The model under review builds one solid part; all positions refer to its coordinate system, in mm. Face numbers are marked on the shaded views. A direction names the side the tool comes from. Coordinates: 2 decimals unless noted, no trailing zeros. Write each loop counter-clockwise with the first axis right and the second up, starting at its lowest first coordinate (ties: lowest second). Pieces come first, ordered by that corner, then holes. Notation, with made-up numbers: (15, -21.5) - (58, -21.5) arc R13 ccw to (58, -16.5) - close; hole circle Ø3 at (40.25, 19). An arc over 180 degrees is marked (long way). Put each result on its own line as item: value.
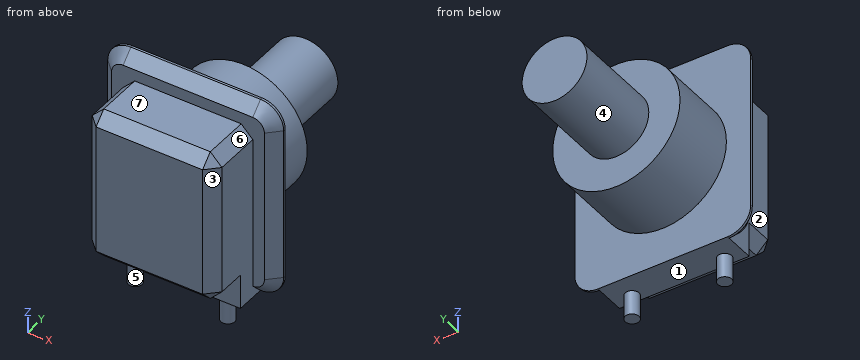
from build123d import *

# Parameters (mm, degrees)
F1_DEPTH  = 6
F2_R      = 27.5
F3_DEPTH  = 30
F4_R      = 14
F5_DEPTH  = 40
F6_W      = 56
F6_H      = 10
F7_DEPTH  = 8
F8_R      = 3
F9_DEPTH  = 10.5
F10_W     = 56
F10_H     = 66
F11_DEPTH = 25
F12_SIZE  = 5


with BuildPart() as f1:
    # F0 (on Front) → F1 (new body)
    with BuildSketch(Plane.XZ):
        with BuildLine():
            ThreePointArc((38, 33), (35.0710678119, 40.0710678119), (28, 43))
            Line((28, 43), (-28, 43))
            ThreePointArc((-28, 43), (-35.0710678119, 40.0710678119), (-38, 33))
            Line((-38, 33), (-38, -33))
            ThreePointArc((-38, -33), (-35.0710678119, -40.0710678119), (-28, -43))
            Line((-28, -43), (28, -43))
            ThreePointArc((28, -43), (35.0710678119, -40.0710678119), (38, -33))
            Line((38, -33), (38, 33))
        make_face()
    extrude(amount=F1_DEPTH)

    # F2 (on face) → F3 (join)
    with BuildSketch(Plane(origin=(0, 0, 0), x_dir=(-1, 0, 0), z_dir=(0, 1, 0))):
        Circle(F2_R)
    extrude(amount=F3_DEPTH)

    # F4 (on face) → F5 (join)
    with BuildSketch(Plane(origin=(0, 30, 0), x_dir=(-1, 0, 0), z_dir=(0, 1, 0))):
        Circle(F4_R)
    extrude(amount=F5_DEPTH)

    # F6 (on face) → F7 (join)
    with BuildSketch(Plane.XZ.offset(6)):
        with Locations((0, -38)):
            Rectangle(F6_W, F6_H)
    extrude(amount=F7_DEPTH)

    # F8 (on face) → F9 (join)
    with BuildSketch(Plane(origin=(0, 0, -43), x_dir=(1, 0, 0), z_dir=(0, 0, -1))):
        with Locations((-20, 10.148444213)):
            Circle(F8_R)
        with Locations((20, 10.148444213)):
            Circle(F8_R)
    extrude(amount=F9_DEPTH)

    # F10 (on face) → F11 (join)
    with BuildSketch(Plane.XZ.offset(6)):
        Rectangle(F10_W, F10_H)
    extrude(amount=F11_DEPTH)

    # F12
    f12_edges = [f1.edges().sort_by_distance(p)[0] for p in [
        (0, -31, 33),
        (28, -31, 0),
        (-28, -31, 0),
        (-28, -18.5, 33),
        (28, -18.5, 33),
        (28, -22.5, -33),
        (0, -31, -33),
        (-28, -22.5, -33),
        (0, -6, 43),
    ]]
    chamfer(f12_edges, length=F12_SIZE)


solid = f1.part
1. Machinability: for the marked faces 4, 5, 6 and 7, which of the approach directions +Z, -Z, +X, -X, +Y, -Y give a long, thin tool a straight path to every point of the face, cutting with its end or side? Answer none if there is none.
Determined:
face 4: +Y
face 5: -Z
face 6: +Z, +X, -Y
face 7: +Z, +X, -X, -Y
2. The part is to be moulded in two halves that separate along X. For the marked faces 1, 2 and 3, say which applies: +X half, -X half, draft (parallel to the pull), parting line (faces both ways), or undercut.
Determined:
face 1: undercut
face 2: -X half
face 3: +X half
3. Consider section D-D on x = 20.5. State the section outline as (y, z) points.
Determined:
outline: (-31, -28) - (-26, -33) - (-14, -33) - (-14, -43) - (-13.11, -43) - (-13.11, -53.5) - (-7.19, -53.5) - (-7.19, -43) - (0, -43) - (0, -18.33) - (30, -18.33) - (30, 18.33) - (0, 18.33) - (0, 43) - (-1, 43) - (-6, 38) - (-6, 33) - (-26, 33) - (-31, 28) - close
4. For pin 1 Ø1.5 at (y, z) = (29, 2.5) entering from +X; pin 2 Ø1 at (y, z) = (20, -14.5) entering from +X; pin 3 Ø8 at (x, y) = (17.5, 22) entering from -Z; pin 4 Ø6 at (x, y) = (19, 52) entering from -Z, all flat-tipped, find the tip position at first contact; note any pin that passes through.
Determined:
pin 1: stops at x = 27.44
pin 2: stops at x = 23.67
pin 3: stops at z = -23.96
pin 4: passes through
5. Consider section A-A on x = 0. State the section outline as (y, z) points.
Determined:
outline: (-31, -28) - (-26, -33) - (-14, -33) - (-14, -43) - (0, -43) - (0, -27.5) - (30, -27.5) - (30, -14) - (70, -14) - (70, 14) - (30, 14) - (30, 27.5) - (0, 27.5) - (0, 43) - (-1, 43) - (-6, 38) - (-6, 33) - (-26, 33) - (-31, 28) - close
6. Consider section C-C on y = 57. State the section outline as (x, z) points, plus the area to 3 significant figures.
Determined:
outline: circle Ø28 at (0, 0)
area: 616 mm^2
7. Consider section B-B on z = 0. State the section outline as (x, y) points.
Determined:
outline: (-38, -1) - (-33, -6) - (-28, -6) - (-28, -26) - (-23, -31) - (23, -31) - (28, -26) - (28, -6) - (33, -6) - (38, -1) - (38, 0) - (27.5, 0) - (27.5, 30) - (14, 30) - (14, 70) - (-14, 70) - (-14, 30) - (-27.5, 30) - (-27.5, 0) - (-38, 0) - close
8. To check wall thickness, follow probe 1 along Y at (x, z) = (16, 16.5); probe 2 along Y at (x, z) = (9.5, -37); probe 3 along X at (y, z) = (-6.5, 1). State the ranges of each line that lie inside material, in increasing order.
Determined:
probe 1: y = -31 to 30
probe 2: y = -14 to 0
probe 3: x = -28 to 28
